```python
from build123d import *

# Parameters (mm, degrees)
F0_W      = 58
F0_H      = 38
F1_DEPTH  = 2
F2_W      = 58
F2_H      = 38
F2_W_2    = 54
F2_H_2    = 34
F3_DEPTH  = 10
F5_W      = 9
F5_H      = 2
F6_DEPTH  = 12.5
F7_R      = 2
F8_R      = 0.5
F9_R      = 1
F10_W     = 10
F10_H     = 2
F11_DEPTH = 58.0010001
F12_SIZE  = 1
F14_R     = 0.5
F15_DEPTH = 25


with BuildPart() as f1:
    # F0 (on Top) → F1 (new body)
    with BuildSketch(Plane.XY):
        with Locations((-18.2900002897, -8.8110647003)):
            Rectangle(F0_W, F0_H)
    extrude(amount=F1_DEPTH)

    # F2 (on face) → F3 (join)
    with BuildSketch(Plane.XY.offset(2)):
        with Locations((-18.2900002897, -8.8110647003)):
            Rectangle(F2_W, F2_H)
        with Locations((-18.2900002897, -8.8110647003)):
            Rectangle(F2_W_2, F2_H_2, mode=Mode.SUBTRACT)
    extrude(amount=F3_DEPTH)

    # F5 (on Top) → F6 (cut, symmetric)
    with BuildSketch(Plane.XY):
        with Locations((-35.7900002897, -20.8110647003)):
            Rectangle(F5_W, F5_H)
        with Locations((-35.7900002897, 3.1889352997)):
            Rectangle(F5_W, F5_H)
        with Locations((-0.7900002897, 3.1889352997)):
            Rectangle(F5_W, F5_H)
        with Locations((-0.7900002897, -20.8110647003)):
            Rectangle(F5_W, F5_H)
    extrude(amount=F6_DEPTH, both=True, mode=Mode.SUBTRACT)

    # F7
    f7_edges = [f1.edges().sort_by_distance(p)[0] for p in [
        (-47.29, -27.811065, 6),
        (10.71, -27.811065, 6),
        (10.71, 10.188935, 6),
        (-47.29, 10.188935, 6),
    ]]
    fillet(f7_edges, radius=F7_R)

    # F8
    f8_edges = [f1.edges().sort_by_distance(p)[0] for p in [
        (-0.79, 2.188935, 2),
        (-0.79, 4.188935, 2),
        (3.71, 3.188935, 2),
        (-5.29, 3.188935, 2),
        (-35.79, 2.188935, 2),
        (-35.79, 4.188935, 2),
        (-31.29, 3.188935, 2),
        (-40.29, 3.188935, 2),
        (-35.79, -19.811065, 2),
        (-35.79, -21.811065, 2),
        (-40.29, -20.811065, 0),
        (-31.29, -20.811065, 2),
        (-40.29, -20.811065, 2),
        (-0.79, -21.811065, 2),
        (-0.79, -19.811065, 2),
        (-5.29, -20.811065, 2),
        (3.71, -20.811065, 2),
    ]]
    fillet(f8_edges, radius=F8_R)

    # F9
    f9_edges = [f1.edges().sort_by_distance(p)[0] for p in [
        (-47.29, -8.811065, 12),
        (-18.29, -27.811065, 12),
        (10.71, -8.811065, 12),
        (-18.29, 10.188935, 12),
        (10.124213, 9.603149, 12),
        (-46.704214, 9.603149, 12),
        (10.124213, -27.225278, 12),
        (-46.704214, -27.225278, 12),
    ]]
    fillet(f9_edges, radius=F9_R)

    # F10 (on face) → F11 (cut, through all)
    with BuildSketch(Plane.YZ.offset(10.7099997103)):
        with Locations((-8.8110647003, 8)):
            Rectangle(F10_W, F10_H)
    extrude(amount=-F11_DEPTH, mode=Mode.SUBTRACT)

    # F12
    f12_edges = [f1.edges().sort_by_distance(p)[0] for p in [
        (-45.29, 8.188935, 7),
        (8.71, 8.188935, 7),
        (-45.29, -25.811065, 7),
        (8.71, -25.811065, 7),
    ]]
    chamfer(f12_edges, length=F12_SIZE)

    # F14 (on face) → F15 (cut)
    with BuildSketch(Plane.XY.offset(2)):
        with Locations((-41.7900002897, 4.6889352997)):
            Circle(F14_R)
        with Locations((5.2099997103, 3.1889352997)):
            Circle(F14_R)
        with Locations((5.2099997103, -17.8110647003)):
            Circle(F14_R)
    extrude(amount=-F15_DEPTH, mode=Mode.SUBTRACT)


solid = f1.part
```
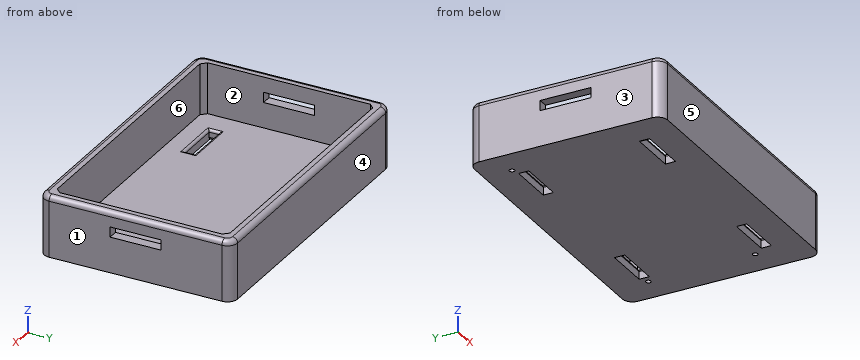
Here's how the part is built. I have some questions about the finished solid (model axes, mm). Face numbers are marked on the shaded views. A direction names the side the tool comes from. Give positions to 0.01 mm unless a question says otherwise; leave off trailing zeros. Order: outer loops, then holes, each group sorted by start corner. A loop starts at its lowest first (then second) coordinate and runs counter-clockwise, first axis right, second up. Notation, with made-up numbers: (10, -28) - (15, -28) arc R31 ccw to (15, 7) - close; hole circle Ø9 at (63.5, 53.25). An arc over 180 degrees is marked (long way). Answer as a JSON object with one key per item and string values. Group by question number.
Item 1: Which directions (+Z, -Z, +X, -X, +Y, -Y) give clear straight access to the entire face, cutting with the end or side of a thin tool? Please do the marked faces 5 and 6.
Item 2: If we section it at B-B on y = -7: Please give me the cut outline in (x, z).
Item 3: If we section it at A-A on z = 9.75: Please give me the cut outline in (x, y).
Item 4: Please list where these lines run through material, in increasing order: probe 1 along Y at (x, z) = (5.21, 1); probe 2 along Y at (x, z) = (-8.5, 4); probe 3 along X at (y, z) = (-22, 3.5).
Item 5: If we mould it in two halves opening along X, with no side actions, what happens to the marked faces 1, 2, 3 and 4? For each: pulls with the +X half, pulls with the -X half, needs draft (parallel to the pull), parting line crosses it, or undercut.
Item 6: If we section it at D-D on y = 1: Please give me the cut outline in (x, z), and give its area (3 significant figures).
Item 7: For P1, Ø0.6, axis at x = 10, z = 8.5, coming from the -Y side; P2, Ø17, axis at x = -19, y = -3, coming from the +Z side; P3, Ø1, axis at x = -46.5, z = 8.5, coming from the -Y side, each with a flat end and sliding along its axis, tell me the tip position at first contact or that it passes through.
Item 8: If we section it at C-C on x = -3: Please give me the cut outline in (y, z), and give its area (3 significant figures).
Result set:
{
 "1": {"face 5": "+Z, -Z, +X, -X, -Y", "face 6": "+Z"},
 "2": {"outline": "(-47.29, 0) - (10.71, 0) - (10.71, 7) - (8.71, 7) - (8.71, 2) - (-45.29, 2) - (-45.29, 7) - (-47.29, 7) - close; (-47.29, 9) - (-45.29, 9) - (-45.29, 12) - (-46.29, 12) arc R1 ccw to (-47.29, 11) - close; (8.71, 9) - (10.71, 9) - (10.71, 11) arc R1 ccw to (9.71, 12) - (8.71, 12) - close"},
 "3": {"outline": "(-47.29, -25.81) arc R2 ccw to (-45.29, -27.81) - (8.71, -27.81) arc R2 ccw to (10.71, -25.81) - (10.71, 8.19) arc R2 ccw to (8.71, 10.19) - (-45.29, 10.19) arc R2 ccw to (-47.29, 8.19) - close; hole (-45.29, -24.81) - (-44.29, -25.81) - (7.71, -25.81) - (8.71, -24.81) - (8.71, 7.19) - (7.71, 8.19) - (-44.29, 8.19) - (-45.29, 7.19) - close"},
 "4": {"probe 1": "-27.81 to -18.31, -17.31 to 2.69, 3.69 to 10.19", "probe 2": "-27.81 to -25.81, 8.19 to 10.19", "probe 3": "-47.29 to -45.29, 8.71 to 10.71"},
 "5": {"face 1": "pulls with the +X half", "face 2": "undercut", "face 3": "pulls with the -X half", "face 4": "needs draft"},
 "6": {"outline": "(-47.29, 0) - (10.71, 0) - (10.71, 11) arc R1 ccw to (9.71, 12) - (8.71, 12) - (8.71, 2) - (-45.29, 2) - (-45.29, 12) - (-46.29, 12) arc R1 ccw to (-47.29, 11) - close", "area": "156 mm²"},
 "7": {"P1": "y = -27.55", "P2": "z = 2", "P3": "y = -27.68"},
 "8": {"outline": "(-27.81, 0) - (-21.81, 0) - (-21.81, 1.5) arc R0.5 ccw to (-22.31, 2) - (-25.81, 2) - (-25.81, 12) - (-26.81, 12) arc R1 ccw to (-27.81, 11) - close; (-19.81, 0) - (2.19, 0) - (2.19, 1.5) arc R0.5 ccw to (1.69, 2) - (-19.31, 2) arc R0.5 ccw to (-19.81, 1.5) - close; (4.19, 0) - (10.19, 0) - (10.19, 11) arc R1 ccw to (9.19, 12) - (8.19, 12) - (8.19, 2) - (4.69, 2) arc R0.5 ccw to (4.19, 1.5) - close", "area": "107 mm²"}
}
